from build123d import *

# Parameters (mm, degrees)
F0_W           = 34
F0_H           = 30
F0_W_2         = 26
F0_H_2         = 22
F1_DEPTH       = 15
F3_D           = 3.7973
F3_DEPTH       = 5
F3_CSINK_D     = 7.7978
F3_CSINK_ANGLE = 82
F3_TIP         = 1.1408240143
F4_R           = 3
F5_R           = 1


with BuildPart() as f1:
    # F0 (on Top) → F1 (new body)
    with BuildSketch(Plane.XY):
        Rectangle(F0_W, F0_H)
        Rectangle(F0_W_2, F0_H_2, mode=Mode.SUBTRACT)
    extrude(amount=F1_DEPTH)

    # F3
    with Locations(Plane.XZ.offset(15)):
        with Locations((0, 7.5)):
            CounterSinkHole(F3_D / 2, F3_CSINK_D / 2, depth=F3_DEPTH, counter_sink_angle=F3_CSINK_ANGLE)
            with Locations((0, 0, -(F3_DEPTH + F3_TIP / 2))):  # 118° drill point
                Cone(0, F3_D / 2, F3_TIP, mode=Mode.SUBTRACT)

    # F4
    f4_edges = [f1.edges().sort_by_distance(p)[0] for p in [
        (-17, -15, 7.5),
        (17, -15, 7.5),
        (17, 15, 7.5),
        (-17, 15, 7.5),
        (0, -15, 15),
        (17, 0, 15),
        (0, 15, 15),
        (-17, 0, 15),
    ]]
    fillet(f4_edges, radius=F4_R)

    # F5
    f5_edges = [f1.edges().sort_by_distance(p)[0] for p in [
        (-13, -11, 7.5),
        (-13, 11, 7.5),
        (13, 11, 7.5),
        (13, -11, 7.5),
    ]]
    fillet(f5_edges, radius=F5_R)


solid = f1.part
Source: CAD feature listing. Evaluate the final solid. Frame: model axes, mm. A direction names the side the tool comes from. Round coordinates to 2 decimals unless told otherwise and drop trailing zeros. Write each loop counter-clockwise with the first axis right and the second up, starting at its lowest first coordinate (ties: lowest second). Pieces come first, ordered by that corner, then holes. Notation, with made-up numbers: M 44.25,-10.5 L 98.25,-10.5 A20 ccw 98.25,-1.5 Z; hole C 66.5,83 d1. An arc over 180 degrees is marked long. One line per item, written item: value. Start each with the question number.
Item 1: Set-up query: faces 4 (the cylindrical face through (12.699, -10.715, 7.605)), 5 (the cylindrical face through (16.14, 14.1, 6.08)). Return all of +Z, -Z, +X, -X, +Y, -Y with unobstructed straight access to the full face (end or side cutting, diameter ignored); none if empty.
Item 2: Section query A-A (x = 0). Return the cut outline in (y, z).
Item 3: Pin query (flat end, axial travel): pin 1 (5 mm diameter, centred on x = 0, z = 7.5, fed in from -Y). Return the tip coordinate at first contact, or that it passes through.
Item 4: Section query B-B (z = 2.5). Return the cut outline in (x, y).
Item 5: Section query C-C (y = 5). Return the cut outline in (x, z), plus the area to 3 significant figures.
Item 6: Section query D-D (z = 7.5). Return the cut outline in (x, y), plus the area to 3 significant figures.
Item 7: Mould query, pull axis X, two halves, no side actions, for faces 1 (the flat face through (0, 15, 6)), 2 (the flat face through (-17, 0, 6)), 3 (the flat face through (2, -11, 7)). Classes: pulls with the +X half, pulls with the -X half, needs draft (parallel to the pull), parting line crosses it, or undercut.
Item 8: Ray query, L1, parallel to X at y = -8.25, z = 9.25; L2, parallel to Z at x = 0, y = -11.45; L3, parallel to Y at x = -10, z = 8.5. Return the intervals inside material, ascending. Write a range as from..to.
Result set:
1. face 4: +Z, -Z
1. face 5: +Z, -Z, +X, +Y
2. outline: M -15,0 L -11,0 L -11,5.6 L -12.7,5.6 L -15,3.6 Z; M -15,11.4 L -12.7,9.4 L -11,9.4 L -11,15 L -12,15 A3 ccw -15,12 Z; M 11,0 L 15,0 L 15,12 A3 ccw 12,15 L 11,15 Z
3. pin 1: stops at y = -13.39
4. outline: M -17,-12 A3 ccw -14,-15 L 14,-15 A3 ccw 17,-12 L 17,12 A3 ccw 14,15 L -14,15 A3 ccw -17,12 Z; hole M -13,-10 A1 ccw -12,-11 L 12,-11 A1 ccw 13,-10 L 13,10 A1 ccw 12,11 L -12,11 A1 ccw -13,10 Z
5. outline: M -17,0 L -13,0 L -13,15 L -14,15 A3 ccw -17,12 Z; M 13,0 L 17,0 L 17,12 A3 ccw 14,15 L 13,15 Z
5. area: 116 mm²
6. outline: M -17,-12 A3 ccw -14,-15 L -3.9,-15 L -1.9,-12.7 L -1.9,-11 L -12,-11 A1 cw -13,-10 L -13,10 A1 cw -12,11 L 12,11 A1 cw 13,10 L 13,-10 A1 cw 12,-11 L 1.9,-11 L 1.9,-12.7 L 3.9,-15 L 14,-15 A3 ccw 17,-12 L 17,12 A3 ccw 14,15 L -14,15 A3 ccw -17,12 Z
6. area: 421 mm²
7. face 1: needs draft
7. face 2: pulls with the -X half
7. face 3: undercut
8. L1: x = -17..-13, 13..17
8. L2: z = 0..5.6, 9.4..15
8. L3: y = -15..-11, 11..15
